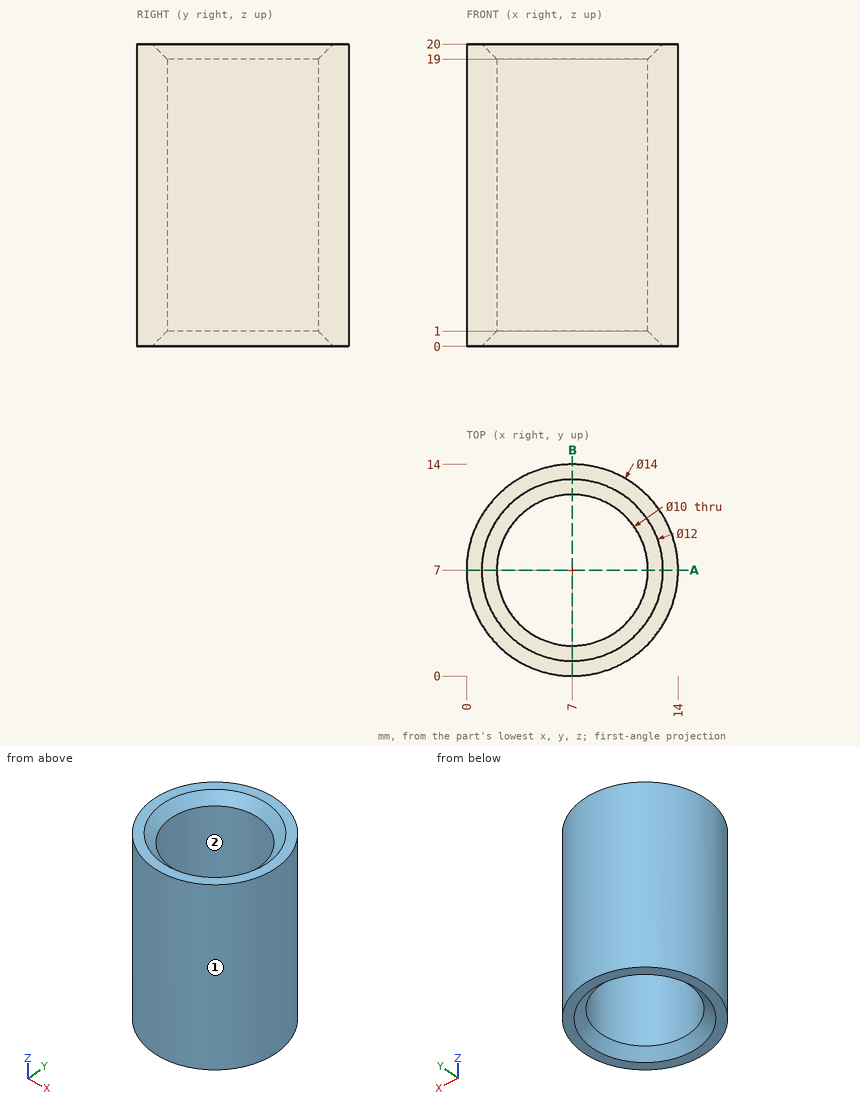
Could you check a few things on this drawing? It's one solid part, dimensions in mm from its lowest x, y, z. Coordinates: 2 decimals unless noted, no trailing zeros. Write each loop counter-clockwise with the first axis right and the second up, starting at its lowest first coordinate (ties: lowest second). Pieces come first, ordered by that corner, then holes.
1) Thinking about a two-plate mould opening in X: for the marked faces 1 and 2, which applies, +X half, -X half, draft (parallel to the pull), parting line (faces both ways), or undercut?
Filled in:
face 1: parting line
face 2: undercut
2) If we section it at A-A (y = 7): List the corners of the cut face in (x, z) for me.
Filled in:
outline: (0, 0) - (1, 0) - (2, 1) - (2, 19) - (1, 20) - (0, 20) - close; (12, 1) - (13, 0) - (14, 0) - (14, 20) - (13, 20) - (12, 19) - close
3) If I drill on line 1 (Y direction, x = 7, z = 15); line 2 (X direction, y = 11.5, z = 5.25); line 3 (Y direction, x = 11, z = 7.5), over which ranges is the centre line in solid material (lowest first)?
Filled in:
line 1: y = 0 to 2, 12 to 14
line 2: x = 1.64 to 4.82, 9.18 to 12.36
line 3: y = 1.26 to 4, 10 to 12.74
4) I'm going to push flat-ended pins straight in: pin 1 (3 mm diameter, centred on x = 5, z = 3, fed in from -Y); pin 2 (3 mm diameter, centred on y = 3, z = 17.5, fed in from +X); pin 3 (3 mm diameter, centred on y = 5, z = 15.5, fed in from +X). Where does each tip first touch, or does it pass through?
Filled in:
pin 1: stops at y = 0.02
pin 2: stops at x = 13.54
pin 3: stops at x = 13.98
